Source: CAD feature listing. Evaluate the final solid. Frame: model axes, mm. Face numbers are marked on the shaded views. A direction names the side the tool comes from. Coordinates: 2 decimals unless noted, no trailing zeros. Order: outer loops, then holes, each group sorted by start corner. A loop starts at its lowest first (then second) coordinate and runs counter-clockwise, first axis right, second up.
Item 1: Section B-B on x = 30.12. Return the cut outline in (y, z) (3 decimals), then the cut area to 3 significant figures.
Item 2: Section D-D on x = 19.96. Return the cut outline in (y, z).
Item 3: Contact query for flat-ended pins moving along their axis: P1, Ø3.5, axis at x = 23, z = -35, coming from the -Y side; P2, Ø2, axis at y = 4, z = -25, coming from the -X side; P3, Ø2.5, axis at x = 19.96, z = -34.8, coming from the +Y side; P4, Ø1.5, axis at x = 14.5, y = 1.5, coming from the -Z side. Output: stop coordinate, or through.
Item 4: Ray query, line 1 (X direction, y = 0.5, z = -11); line 2 (X direction, y = 5.85, z = -34.8); line 3 (Z direction, x = 19.96, y = 4.75). Return the intervals inside material, ascending.
Item 5: Mould query, pull axis Z, two halves, no side actions, for the marked faces 6, 7 and 8. Classes: released by +Z, released by -Z, zero draft, split by the parting line, or undercut.
Item 6: Reachability of the marked faces 1, 2, 3, 4 and 5 from +Z, -Z, +X, -X, +Y, -Y: full face, straight path, thin tool, end or side. Return the list, or none.
Item 7: Section A-A on z = -34.8. Return the cut outline in (x, y).
Item 8: Section C-C on y = 1.5. Return the cut outline in (x, z) (3 decimals).
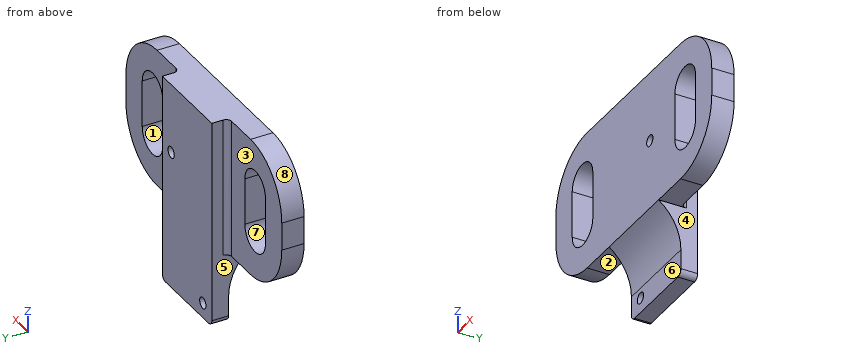
from build123d import *

# Parameters (mm, degrees)
SKETCH1_W                = 50
SKETCH1_H                = 25
BOSS_EXTRUDE1_DEPTH      = 4
SKETCH2_W                = 15.88
SKETCH2_H                = 37.5
BOSS_EXTRUDE2_DEPTH      = 3
M6_CLEARANCE_SLOT1_DEPTH = 4
M3_CLEARANCE_HOLE1_D     = 2
FILLET3_R                = 10
FILLET4_R                = 10
FILLET5_R                = 1


# Read off the part's stored shape, not the designer's step: M6 Clearance Slot1
with BuildPart() as part:
    # Sketch1 → Boss-Extrude1 (new body)
    with BuildSketch(Plane(origin=(0, 0, 0), x_dir=(1, 0, 0), z_dir=(0, 1, 0))):
        with Locations((25, 12.5)):
            Rectangle(SKETCH1_W, SKETCH1_H)
    extrude(amount=BOSS_EXTRUDE1_DEPTH)

    # Sketch2 → Boss-Extrude2 (add)
    with BuildSketch(Plane(origin=(0, 4, 0), x_dir=(1, 0, 0), z_dir=(0, 1, 0))):
        with Locations((25, 18.75)):
            Rectangle(SKETCH2_W, SKETCH2_H)
    extrude(amount=BOSS_EXTRUDE2_DEPTH)

    # M6 Clearance Slot1 outline → M6 Clearance Slot1 (cut)
    with BuildSketch(Plane(origin=(0, 0, 0), x_dir=(1, 0, 0), z_dir=(0, 1, 0))):
        with BuildLine():
            Line((44.77, 8.3), (44.77, 16.7))
            ThreePointArc((44.77, 16.7), (41.47, 20), (38.17, 16.7))
            Line((38.17, 16.7), (38.17, 8.3))
            ThreePointArc((38.17, 8.3), (41.47, 5), (44.77, 8.3))
        make_face()
        with BuildLine():
            Line((11.83, 8.3), (11.83, 16.7))
            ThreePointArc((11.83, 16.7), (8.53, 20), (5.23, 16.7))
            Line((5.23, 16.7), (5.23, 8.3))
            ThreePointArc((5.23, 8.3), (8.53, 5), (11.83, 8.3))
        make_face()
    extrude(amount=M6_CLEARANCE_SLOT1_DEPTH, mode=Mode.SUBTRACT)

    # M3 Clearance Hole1 (through all)
    with Locations(Plane(origin=(0, 7, 0), x_dir=(1, 0, 0), z_dir=(0, 1, 0))):
        with Locations((19.96, 34.8), (30.12, 12.525)):
            Hole(M3_CLEARANCE_HOLE1_D / 2)

    # Fillet3
    fillet3_edges = [part.edges().sort_by_distance(p)[0] for p in [
        (0, 2, -25),
        (50, 2, -25),
        (50, 2, 0),
        (0, 2, 0),
    ]]
    fillet(fillet3_edges, radius=FILLET3_R)

    # Fillet4
    # the kernel refuses this fillet: 10 mm, written as the material it adds along each edge
    with BuildSketch(Plane(origin=(32.94, 4, -25), x_dir=(0, -1, 0), z_dir=(-1, 0, 0))) as fillet4_piece_1:
        with BuildLine():
            CenterArc((10, -8), FILLET4_R, 126.869897646, 53.130102354)
            Line((0, -8), (-0.2, -8))
            Line((-0.2, -8), (-0.2, 0))
            Line((-0.2, 0), (0, 0.2))
            ThreePointArc((0, 0.2), (2, 0.2), (3.88, 0.16))
            Line((3.88, 0.16), (4, 0))
        make_face()
    extrude(amount=15.88)

    # Fillet5
    fillet5_edges = [part.edges().sort_by_distance(p)[0] for p in [
        (32.94, 4, -12.5),
        (17.06, 4, -12.5),
        (32.94, 5.5, -37.5),
        (17.06, 5.5, -37.5),
    ]]
    fillet(fillet5_edges, radius=FILLET5_R)


solid = part.part
Answer list:
1. outline: (0, -25) arc R10 cw to (4, -33) - (4, -37.5) - (7, -37.5) - (7, -13.525) - (0, -13.525) - close; (0, -11.525) - (7, -11.525) - (7, 0) - (0, 0) - close
1. area: 208 mm2
2. outline: (0, -25) arc R10 cw to (4, -33) - (4, -33.8) - (7, -33.8) - (7, 0) - (0, 0) - close; (4, -37.5) - (7, -37.5) - (7, -35.8) - (4, -35.8) - close
3. P1: stops at y = 4
3. P2: stops at x = 5.64
3. P3: stops at y = 7
3. P4: stops at z = -25
4. line 1: x = 0 to 5.23, 11.83 to 38.17, 44.77 to 50
4. line 2: x = 17.06 to 18.96, 20.96 to 32.94
4. line 3: z = -37.5 to -35.8, -33.8 to 0
5. face 6: zero draft
5. face 7: undercut
5. face 8: released by +Z
6. face 1: +Y, -Y
6. face 2: -Z, -X, +Y, -Y
6. face 3: +Z, -Z, -X, +Y
6. face 4: -Z, +X, +Y
6. face 5: -Z, -X, +Y
7. outline: (17.06, 4) - (18.96, 4) - (18.96, 7) - (17.06, 7) - close; (20.96, 4) - (32.94, 4) - (32.94, 7) - (20.96, 7) - close
8. outline: (0, -15) arc R10 ccw to (10, -25) - (17.06, -25) - (17.06, -26.386) - (32.94, -26.386) - (32.94, -25) - (40, -25) arc R10 ccw to (50, -15) - (50, -10) arc R10 ccw to (40, 0) - (10, 0) arc R10 ccw to (0, -10) - close; hole (5.23, -16.7) arc R3.3 ccw to (11.83, -16.7) - (11.83, -8.3) arc R3.3 ccw to (5.23, -8.3) - close; hole circle Ø2 at (30.12, -12.525); hole (38.17, -16.7) arc R3.3 ccw to (44.77, -16.7) - (44.77, -8.3) arc R3.3 ccw to (38.17, -8.3) - close
